Verification items for the finished model (mm, model axes). A direction names the side the tool comes from. Round coordinates to 2 decimals unless told otherwise and drop trailing zeros. Order: outer loops, then holes, each group sorted by start corner. A loop starts at its lowest first (then second) coordinate and runs counter-clockwise, first axis right, second up. Notation, with made-up numbers: (60.25, -33) -> (112.25, -33) arc R14 cw to (112.25, -18) -> close; hole circle Ø3 at (83.25, -15.5). An arc over 180 degrees is marked (long way). Return JSON: item names as keys, results as strings. Group by question number.
Item 1: Draft check along X on faces 6 (the flat face through (576.166, 305, 1)), 7 (the cylindrical face through (570.17, 349.91, 1.48)), 8 (the flat face through (570, 352, 3)), 9 (the flat face through (569.166, 397, 1)). Enter one of: pulls with the +X half, pulls with the -X half, needs draft (parallel to the pull), parting line crosses it, or undercut.
Item 2: Sectioned sample at B-B on z = 1.3. Give the number of separate pieces and of enclosed holes in the cut face, plus the area to 3 significant figures.
Item 3: Sectioned sample at A-A on x = 561. Record the cut outline in (y, z).
Item 4: Access from +Z, -Z, +X, -X, +Y, -Y to the whole of each face (thin tool, end or side, straight path). Record for faces 1 (the flat face through (562, 395.688, 1)), 2 (the flat face through (581, 306.688, 1)), 3 (the flat face through (581.166, 397, 1)), 4 (the flat face through (575, 398.688, 1)), 5 (the flat face through (564.166, 305, 1)).
Item 5: Depth check by flat-ended pin: pin 1 Ø3 at (x, y) = (564, 323) entering from -Z; pin 2 Ø8 at (x, y) = (575.17, 389.69) entering from -Z; pin 3 Ø1.5 at (x, z) = (582.5, 2) entering from +Y; pin 4 Ø0.9 at (y, z) = (397.5, 2) entering from -X. Enter the tip coordinate at first touch or a pass-through.
Item 6: Scan lines: probe 1 along X at (y, z) = (389.5, 2.25); probe 2 along Y at (x, z) = (577.5, 2.3); probe 3 along Y at (x, z) = (582, 0.35). Record each from-to range of solid material in increasing order. Write a range as from..to.
```python
from build123d import *

# Parameters (mm, degrees)
SKETCH_1_R      = 5
SKETCH_1_RX     = 10
SKETCH_1_RY     = 3.757052079
EXTRUDE_1_DEPTH = 3


with BuildPart() as part:
    # 草图1 → 凸台-拉伸1 (new body)
    with BuildSketch(Plane.XY):
        Polygon((555.166453787, 395.688275275), (555.166453787, 306.688275275), (564.166453787, 306.688275275), (564.166453787, 303.688275275), (576.166453787, 303.688275275), (576.166453787, 306.688275275), (585.166453787, 306.688275275), (585.166453787, 395.688275275), (581.166453787, 395.688275275), (581.166453787, 398.688275275), (569.166453787, 398.688275275), (569.166453787, 395.688275275), align=None)
        with Locations((575.166453787, 389.688275275)):
            Circle(SKETCH_1_R, mode=Mode.SUBTRACT)
        with Locations((575.166453787, 349.688275275)):
            Circle(SKETCH_1_R, mode=Mode.SUBTRACT)
        with Locations(Location((575.166453787, 369.688275275), (0, 0, 90))):
            Ellipse(SKETCH_1_RX, SKETCH_1_RY, mode=Mode.SUBTRACT)
    extrude(amount=EXTRUDE_1_DEPTH)


solid = part.part
```
Recorded:
{
 "1": {"face 6": "pulls with the +X half", "face 7": "undercut", "face 8": "needs draft", "face 9": "pulls with the -X half"},
 "2": {"separate pieces": "1", "enclosed holes": "3", "area": "2,470 mm²"},
 "3": {"outline": "(306.69, 0) -> (395.69, 0) -> (395.69, 3) -> (306.69, 3) -> close"},
 "4": {"face 1": "+Z, -Z, -X, +Y", "face 2": "+Z, -Z, +X, -Y", "face 3": "+Z, -Z, +X, +Y", "face 4": "+Z, -Z, +X, -X, +Y", "face 5": "+Z, -Z, -X, -Y"},
 "5": {"pin 1": "z = 0", "pin 2": "through", "pin 3": "y = 395.69", "pin 4": "x = 569.17"},
 "6": {"probe 1": "555.17..570.17, 580.16..585.17", "probe 2": "306.69..345.27, 354.11..361.85, 377.53..385.27, 394.11..398.69", "probe 3": "306.69..395.69"}
}
